Part model, mm, in its own coordinate system. A direction names the side the tool comes from. Coordinates: 2 decimals unless noted, no trailing zeros. Order: outer loops, then holes, each group sorted by start corner. A loop starts at its lowest first (then second) coordinate and runs counter-clockwise, first axis right, second up. Notation, with made-up numbers: M 67.5,45.5 L 83.5,45.5 A22 ccw 83.5,65.5 Z; hole C -31,88.25 d4. An arc over 180 degrees is marked long. Answer in a Markdown table with one row per item. Add a question column.
from build123d import *

# Parameters (mm, degrees)
SKETCH_1_R          = 1.6
EXTRUDE_1_DEPTH     = 3
FILLET_1_R          = 2
CUT_EXTRUDE_1_DEPTH = 10


with BuildPart() as part:
    # 草图1 → 凸台-拉伸1 (new body)
    with BuildSketch(Plane.XY):
        Polygon((0, 0), (28, 0), (58, 30), (58, 58), (50, 58), (0, 8), align=None)
        with Locations((5, 6)):
            Circle(SKETCH_1_R, mode=Mode.SUBTRACT)
        with Locations((25, 6)):
            Circle(SKETCH_1_R, mode=Mode.SUBTRACT)
        with Locations(Location((52, 53, 0), (0, 0, 180))):
            Circle(SKETCH_1_R, mode=Mode.SUBTRACT)
        with Locations(Location((52, 33, 0), (0, 0, 180))):
            Circle(SKETCH_1_R, mode=Mode.SUBTRACT)
    extrude(amount=EXTRUDE_1_DEPTH)

    # 圆角1
    fillet_1_edges = [part.edges().sort_by_distance(p)[0] for p in [
        (0, 8, 1.5),
        (50, 58, 1.5),
        (58, 58, 1.5),
        (58, 30, 1.5),
        (28, 0, 1.5),
        (0, 0, 1.5),
    ]]
    fillet(fillet_1_edges, radius=FILLET_1_R)

    # 草图2 → 切除-拉伸1 (cut)
    with BuildSketch(Plane.XY.offset(3)):
        with BuildLine():
            Line((10.857864376, 13.201010127), (25, 27.343145751))
            ThreePointArc((25, 27.343145751), (27.828427125, 27.343145751), (27.828427125, 24.514718626))
            Line((27.828427125, 24.514718626), (13.686291501, 10.372583002))
            ThreePointArc((13.686291501, 10.372583002), (10.857864376, 10.372583002), (10.857864376, 13.201010127))
        make_face()
        with BuildLine():
            Line((32.778174593, 19.564971157), (23.585786438, 10.372583002))
            ThreePointArc((23.585786438, 10.372583002), (20.757359313, 10.372583002), (20.757359313, 13.201010127))
            Line((20.757359313, 13.201010127), (29.949747468, 22.393398282))
            ThreePointArc((29.949747468, 22.393398282), (32.778174593, 22.393398282), (32.778174593, 19.564971157))
        make_face()
        with BuildLine():
            Line((30.656854249, 13.201010127), (34.899494937, 17.443650814))
            ThreePointArc((34.899494937, 17.443650814), (37.727922061, 17.443650814), (37.727922061, 14.615223689))
            Line((37.727922061, 14.615223689), (33.485281374, 10.372583002))
            ThreePointArc((33.485281374, 10.372583002), (30.656854249, 10.372583002), (30.656854249, 13.201010127))
        make_face()
        with BuildLine():
            Line((44.798989873, 47.142135624), (30.656854249, 33))
            ThreePointArc((30.656854249, 33), (30.656854249, 30.171572875), (33.485281374, 30.171572875))
            Line((33.485281374, 30.171572875), (47.627416998, 44.313708499))
            ThreePointArc((47.627416998, 44.313708499), (47.627416998, 47.142135624), (44.798989873, 47.142135624))
        make_face()
        with BuildLine():
            Line((38.435028843, 25.221825407), (47.627416998, 34.414213562))
            ThreePointArc((47.627416998, 34.414213562), (47.627416998, 37.242640687), (44.798989873, 37.242640687))
            Line((44.798989873, 37.242640687), (35.606601718, 28.050252532))
            ThreePointArc((35.606601718, 28.050252532), (35.606601718, 25.221825407), (38.435028843, 25.221825407))
        make_face()
        with BuildLine():
            Line((44.798989873, 27.343145751), (40.556349186, 23.100505063))
            ThreePointArc((40.556349186, 23.100505063), (40.556349186, 20.272077939), (43.384776311, 20.272077939))
            Line((43.384776311, 20.272077939), (47.627416998, 24.514718626))
            ThreePointArc((47.627416998, 24.514718626), (47.627416998, 27.343145751), (44.798989873, 27.343145751))
        make_face()
    extrude(amount=-CUT_EXTRUDE_1_DEPTH, mode=Mode.SUBTRACT)


solid = part.part
(1) 3-axis set-ups, long thin cutter, end or side, ignore diameter. For faces 4 (the flat face through (53, 58, 1)), 5 (the flat face through (17.83, 20.173, 1.521)): which of +Z, -Z, +X, -X, +Y, -Y reach the whole face in a straight line?
(2) Drop flat-ended pins along their axis: P1, Ø1.5, axis at y = 31.5, z = 2.5, coming from the -X side; P2, Ø2.5, axis at x = 25, y = 6, coming from the -Z side; P3, Ø1, axis at x = 37, z = 2.5, coming from the +Y side. Give the stop position or say it passes through.
(3) Slice it at C-C (y = 53). List the corners of the cut face in (x, z).
(4) Wall check: line 1 (Y direction, x = 21, z = 2.8); line 2 (Y direction, x = 43, z = 0.95); line 3 (X direction, y = 33, z = 0.75). Give the ranges that are in metal, low to high.
(5) Slice it at B-B (y = 6). List the corners of the cut face in (x, z), and give its area (3 significant figures).
(6) Slice it at A-A (x = 52). List the corners of the cut face in (y, z).
(7) Pull direction X, two halves, no side cores. Call faces 1 (the flat face through (14, 0, 1)), 2 (the flat face through (40.267, 32.711, 1.521)), 3 (the flat face through (0, 5, 1)): pulls with the +X half, pulls with the -X half, needs draft (parallel to the pull), parting line crosses it, or undercut.
(8) Slice it at D-D (x = 5). List the corners of the cut face in (y, z).
Computed:
| question | item | result |
|---|---|---|
| 1 | face 4 | +Z, -Z, +X, -X, +Y |
| 1 | face 5 | +Z, -Z |
| 2 | P1 | stops at x = 22.75 |
| 2 | P2 | passes through |
| 2 | P3 | stops at y = 45.5 |
| 3 | outline | M 45,0 L 50.4,0 L 50.4,3 L 45,3 Z; M 53.6,0 L 58,0 L 58,3 L 53.6,3 Z |
| 4 | line 1 | y = 0 to 10.17, 13.44 to 17.69, 23.34 to 29 |
| 4 | line 2 | y = 15 to 19.97, 25.54 to 29.79, 35.44 to 39.69, 45.34 to 51 |
| 4 | line 3 | x = 25 to 30.66, 36.31 to 40.56, 46.21 to 50.4, 53.6 to 58 |
| 5 | outline | M 0,0 L 3.4,0 L 3.4,3 L 0,3 Z; M 6.6,0 L 23.4,0 L 23.4,3 L 6.6,3 Z; M 26.6,0 L 34,0 L 34,3 L 26.6,3 Z |
| 5 | area | 82.8 mm^2 |
| 6 | outline | M 24,0 L 31.4,0 L 31.4,3 L 24,3 Z; M 34.6,0 L 51.4,0 L 51.4,3 L 34.6,3 Z; M 54.6,0 L 58,0 L 58,3 L 54.6,3 Z |
| 7 | face 1 | needs draft |
| 7 | face 2 | undercut |
| 7 | face 3 | pulls with the -X half |
| 8 | outline | M 0,0 L 4.4,0 L 4.4,3 L 0,3 Z; M 7.6,0 L 13,0 L 13,3 L 7.6,3 Z |
